The listing builds one solid part. Answer for the finished solid, in the listing's coordinates (mm). Face numbers are marked on the shaded views. A direction names the side the tool comes from. Give positions to 0.01 mm unless a question says otherwise; leave off trailing zeros. Order: outer loops, then holes, each group sorted by start corner. A loop starts at its lowest first (then second) coordinate and runs counter-clockwise, first axis right, second up.
```python
from build123d import *

# Parameters (mm, degrees)
BOX002_W     = 10
BOX002_H     = 10
BOX002_DEPTH = 10
BOX003_W     = 20
BOX003_H     = 10
BOX003_DEPTH = 10
BOX004_W     = 10
BOX004_H     = 20
BOX004_DEPTH = 10
BOX_W        = 20
BOX_H        = 30
BOX_DEPTH    = 10


with BuildPart() as cubo002:
    # Box002 → Box002 (new body)
    with BuildSketch(Plane(origin=(0, 20, 20), x_dir=(1, 0, 0), z_dir=(0, 0, 1))):
        with Locations((5, 5)):
            Rectangle(BOX002_W, BOX002_H)
    extrude(amount=BOX002_DEPTH)


with BuildPart() as cubo003:
    # Box003 → Box003 (new body)
    with BuildSketch(Plane(origin=(0, 20, 10), x_dir=(1, 0, 0), z_dir=(0, 0, 1))):
        with Locations((10, 5)):
            Rectangle(BOX003_W, BOX003_H)
    extrude(amount=BOX003_DEPTH)


with BuildPart() as cubo004:
    # Box004 → Box004 (new body)
    with BuildSketch(Plane(origin=(20, 10, 0), x_dir=(1, 0, 0), z_dir=(0, 0, 1))):
        with Locations((5, 10)):
            Rectangle(BOX004_W, BOX004_H)
    extrude(amount=BOX004_DEPTH)


with BuildPart() as fusion:
    # Box → Box (new body)
    with BuildSketch(Plane.XY):
        with Locations((10, 15)):
            Rectangle(BOX_W, BOX_H)
    extrude(amount=BOX_DEPTH)

    # Fusion: union Cubo002, Cubo003, Cubo004
    add(cubo002.part)
    add(cubo003.part)
    add(cubo004.part)


solid = fusion.part
```
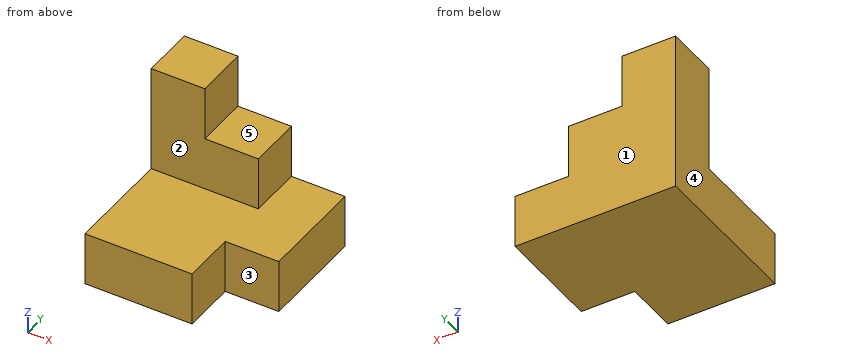
1) Find section A-A (y = 22). Write down the section's boundary in (x, z), then the cut area to 3 significant figures.
Geometry says:
outline: (0, 0) - (30, 0) - (30, 10) - (20, 10) - (20, 20) - (10, 20) - (10, 30) - (0, 30) - close
area: 600 mm2
2) Straight lines are drawn through the part: probe 1 along Y at (x, z) = (9, 20.25); probe 2 along Z at (x, y) = (23.5, 17.75); probe 3 along X at (y, z) = (25.5, 11). For each, find the intervals that lie inside material, in ascending order.
Geometry says:
probe 1: y = 20 to 30
probe 2: z = 0 to 10
probe 3: x = 0 to 20
3) Find section B-B (z = 9). Write down the section's boundary in (x, y).
Geometry says:
outline: (0, 0) - (20, 0) - (20, 10) - (30, 10) - (30, 30) - (0, 30) - close
4) A tool of negligible diameter and unlimited length cuts with its end or side. For the marked faces 1, 2, 3, 4 and 5, from which of +Z, -Z, +X, -X, +Y, -Y can it reach the whole face along a straight path? Write none if from no direction.
Geometry says:
face 1: +Z, -Z, +X, -X, +Y
face 2: +Z, +X, -X, -Y
face 3: +Z, -Z, +X, -Y
face 4: +Z, -Z, -X, +Y, -Y
face 5: +Z, +X, +Y, -Y
5) Find section C-C (x = 8). Write down the section's boundary in (y, z).
Geometry says:
outline: (0, 0) - (30, 0) - (30, 30) - (20, 30) - (20, 10) - (0, 10) - close
6) Find section D-D (y = 4.5). Write down the section's boundary in (x, z).
Geometry says:
outline: (0, 0) - (20, 0) - (20, 10) - (0, 10) - close
7) Given P1, Ø8, axis at y = 2.5, z = 7, coming from the +X side; P2, Ø6, axis at x = 12.5, z = 26.5, coming from the +Y side; P3, Ø2, axis at x = 27, y = 18.5, coming from the +Z side; P4, Ø10, axis at x = 5, z = 22.5, coming from the -Y side, each flat-ended and moving along its own axis, determine where each tip first touches the part or whether it passes through.
Geometry says:
P1: stops at x = 20
P2: stops at y = 30
P3: stops at z = 10
P4: stops at y = 20
